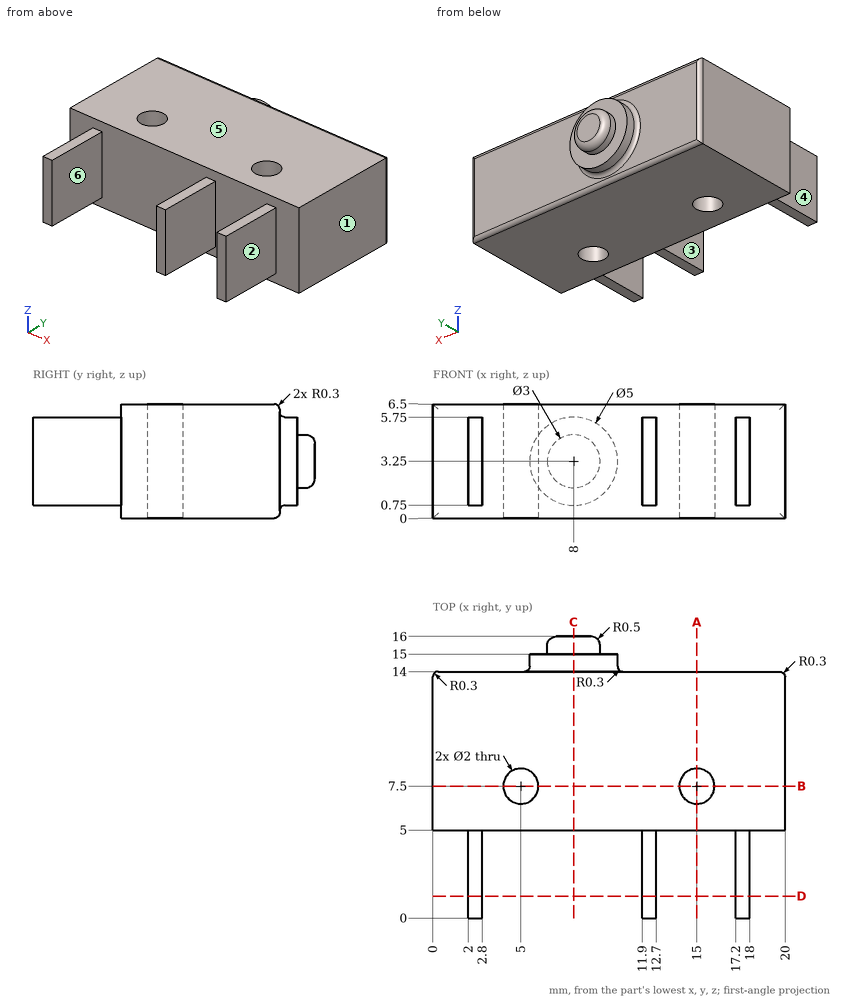
Design review of the part shown in the three views and the two pictorial views. Dimensions are in mm from the part's minimum x, y and z. A direction names the side the tool comes from. Give positions to 0.01 mm unless a question says otherwise; leave off trailing zeros. Write each loop counter-clockwise with the first axis right and the second up, starting at its lowest first coordinate (ties: lowest second). Pieces come first, ordered by that corner, then holes. Notation, with made-up numbers: (82, 85.25) - (112, 85.25) arc R26 ccw to (112, 102.25) - close; hole circle Ø8 at (29, 49). An arc over 180 degrees is marked (long way). Return JSON: item names as keys, results as strings. Group by question number.
(1) Mouldability with a two-part tool opening along X and no side actions: class the marked faces 4, 5 and 6 as +X half, -X half, draft (parallel to the pull), parting line (faces both ways), or undercut.
(2) Machinability: for the marked faces 1, 2 and 3, which of the approach directions +Z, -Z, +X, -X, +Y, -Y give a long, thin tool a straight path to every point of the face, cutting with its end or side? Answer none if there is none.
(3) To check wall thickness, follow probe 1 along X at (y, z) = (2.25, 4.75); probe 2 along Y at (x, z) = (5, 1.5); probe 3 along Y at (x, z) = (8, 1.5). State the ranges of each line that lie inside material, in increasing order.
(4) We need section B-B, the plane y = 7.5. Give the boundary of the cut face in (x, z).
(5) We need section C-C, the plane x = 8. Give the boundary of the cut face in (y, z), then the cut area to 3 significant figures.
(6) We need section A-A, the plane x = 15. Give the boundary of the cut face in (y, z), then the cut area to 3 significant figures.
(7) Insertion check: pin 1 (0.9 mm diameter, centred on x = 12.5, y = 1.5, fed in from +Z); pin 2 (3 mm diameter, centred on y = 4.5, z = 1.5, fed in from +X); pin 3 (0.6 mm diameter, centred on x = 12, y = 3.5, fed in from -Z); pin 4 (1.8 mm diameter, centred on x = 5, y = 7.5, fed in from +Z). Each pin has a flat end and moves straight along its axis. Give the tip position at first contact, or say it passes through.
(8) We need section D-D, the plane y = 1.25. Give the boundary of the cut face in (x, z).
Reported:
{
 "1": {"face 4": "-X half", "face 5": "draft", "face 6": "undercut"},
 "2": {"face 1": "+Z, -Z, +X, +Y, -Y", "face 2": "+Z, -Z, +X, -Y", "face 3": "+Z, -Z, -Y"},
 "3": {"probe 1": "x = 2 to 2.8, 11.9 to 12.7, 17.2 to 18", "probe 2": "y = 5 to 6.5, 8.5 to 14", "probe 3": "y = 5 to 15"},
 "4": {"outline": "(0, 0) - (4, 0) - (4, 6.5) - (0, 6.5) - close; (6, 0) - (14, 0) - (14, 6.5) - (6, 6.5) - close; (16, 0) - (20, 0) - (20, 6.5) - (16, 6.5) - close"},
 "5": {"outline": "(5, 0) - (13.7, 0) arc R0.3 ccw to (14, 0.3) - (14, 0.45) arc R0.3 cw to (14.3, 0.75) - (15, 0.75) - (15, 1.75) - (15.5, 1.75) arc R0.5 ccw to (16, 2.25) - (16, 4.25) arc R0.5 ccw to (15.5, 4.75) - (15, 4.75) - (15, 5.75) - (14.3, 5.75) arc R0.3 cw to (14, 6.05) - (14, 6.2) arc R0.3 ccw to (13.7, 6.5) - (5, 6.5) - close", "area": "66.4 mm2"},
 "6": {"outline": "(5, 0) - (6.5, 0) - (6.5, 6.5) - (5, 6.5) - close; (8.5, 0) - (13.7, 0) arc R0.3 ccw to (14, 0.3) - (14, 6.2) arc R0.3 ccw to (13.7, 6.5) - (8.5, 6.5) - close", "area": "45.5 mm2"},
 "7": {"pin 1": "stops at z = 5.75", "pin 2": "stops at x = 20", "pin 3": "stops at z = 0.75", "pin 4": "passes through"},
 "8": {"outline": "(2, 0.75) - (2.8, 0.75) - (2.8, 5.75) - (2, 5.75) - close; (11.9, 0.75) - (12.7, 0.75) - (12.7, 5.75) - (11.9, 5.75) - close; (17.2, 0.75) - (18, 0.75) - (18, 5.75) - (17.2, 5.75) - close"}
}
